from build123d import *

# Parameters (mm, degrees)
SKETCH1_R           = 2.0999999
BOSS_EXTRUDE1_DEPTH = 420


with BuildPart() as part:
    # Sketch1 → Boss-Extrude1 (new body)
    with BuildSketch(Plane.XY):
        with BuildLine():
            Line((-10, -13.3000005), (-10, -19))
            ThreePointArc((-10, -19), (-9.707106781, -19.707106781), (-9, -20))
            Line((-9, -20), (-3.3, -20))
            ThreePointArc((-3.3, -20), (-3.087867966, -19.912132034), (-3, -19.7))
            Line((-3, -19.7), (-3, -18))
            Line((-3, -18), (-6, -18))
            Line((-6, -18), (-6, -17.0606825))
            Line((-6, -17.0606825), (-2.939318, -14))
            Line((-2.939318, -14), (-0.519615242, -14))
            Line((-0.519615242, -14), (0, -13.7))
            Line((0, -13.7), (0.519615242, -14))
            Line((0.519615242, -14), (2.9393365, -14))
            Line((2.9393365, -14), (6, -17.0606628))
            Line((6, -17.0606628), (6, -18))
            Line((6, -18), (3, -18))
            Line((3, -18), (3, -19.7))
            ThreePointArc((3, -19.7), (3.087867966, -19.912132034), (3.3, -20))
            Line((3.3, -20), (9, -20))
            ThreePointArc((9, -20), (9.707106781, -19.707106781), (10, -19))
            Line((10, -19), (10, -13.3000005))
            ThreePointArc((10, -13.3000005), (9.912132034, -13.087868466), (9.7, -13.0000005))
            Line((9.7, -13.0000005), (8, -13.0000005))
            Line((8, -13.0000005), (8, -16.0000005))
            Line((8, -16.0000005), (7.06065685, -16.0000005))
            Line((7.06065685, -16.0000005), (4, -12.93934215))
            Line((4, -12.93934215), (4, -10.519615742))
            Line((4, -10.519615742), (3.7, -10.0000005))
            Line((3.7, -10.0000005), (4, -9.480385258))
            Line((4, -9.480385258), (4, -7.06068365))
            Line((4, -7.06068365), (7.06068236, -4.000000504))
            Line((7.06068236, -4.000000504), (8, -4.000000504))
            Line((8, -4.000000504), (8, -7.0000005))
            Line((8, -7.0000005), (9.7, -7.0000005))
            ThreePointArc((9.7, -7.0000005), (9.912132034, -6.912132534), (10, -6.7000005))
            Line((10, -6.7000005), (10, 6.7))
            ThreePointArc((10, 6.7), (9.912132034, 6.912132034), (9.7, 7))
            Line((9.7, 7), (8, 7))
            Line((8, 7), (8, 4))
            Line((8, 4), (7.060678, 4))
            Line((7.060678, 4), (4, 7.06068075))
            Line((4, 7.06068075), (4, 9.480384758))
            Line((4, 9.480384758), (3.7, 10))
            Line((3.7, 10), (4, 10.519615242))
            Line((4, 10.519615242), (4, 12.93933675))
            Line((4, 12.93933675), (7.060661, 16))
            Line((7.060661, 16), (8, 16))
            Line((8, 16), (8, 13))
            Line((8, 13), (9.7, 13))
            ThreePointArc((9.7, 13), (9.912132034, 13.087867966), (10, 13.3))
            Line((10, 13.3), (10, 19))
            ThreePointArc((10, 19), (9.707106781, 19.707106781), (9, 20))
            Line((9, 20), (3.3, 20))
            ThreePointArc((3.3, 20), (3.087867966, 19.912132034), (3, 19.7))
            Line((3, 19.7), (3, 18))
            Line((3, 18), (6, 18))
            Line((6, 18), (6, 17.06065975))
            Line((6, 17.06065975), (2.939354, 14))
            Line((2.939354, 14), (0.519638625, 14))
            Line((0.519638625, 14), (0, 13.6999865))
            Line((0, 13.6999865), (-0.519638625, 14))
            Line((-0.519638625, 14), (-2.939335, 14))
            Line((-2.939335, 14), (-6, 17.060678))
            Line((-6, 17.060678), (-6, 18))
            Line((-6, 18), (-3, 18))
            Line((-3, 18), (-3, 19.7))
            ThreePointArc((-3, 19.7), (-3.087867966, 19.912132034), (-3.3, 20))
            Line((-3.3, 20), (-9, 20))
            ThreePointArc((-9, 20), (-9.707106781, 19.707106781), (-10, 19))
            Line((-10, 19), (-10, 13.3))
            ThreePointArc((-10, 13.3), (-9.912132034, 13.087867966), (-9.7, 13))
            Line((-9.7, 13), (-8, 13))
            Line((-8, 13), (-8, 16))
            Line((-8, 16), (-7.060642, 16))
            Line((-7.060642, 16), (-4, 12.9393565))
            Line((-4, 12.9393565), (-4, 10.519615242))
            Line((-4, 10.519615242), (-3.7, 10))
            Line((-3.7, 10), (-4, 9.480384758))
            Line((-4, 9.480384758), (-4, 7.06066))
            Line((-4, 7.06066), (-7.060659, 4))
            Line((-7.060659, 4), (-8, 4))
            Line((-8, 4), (-8, 7))
            Line((-8, 7), (-9.7, 7))
            ThreePointArc((-9.7, 7), (-9.912132034, 6.912132034), (-10, 6.7))
            Line((-10, 6.7), (-10, -6.7000005))
            ThreePointArc((-10, -6.7000005), (-9.912132034, -6.912132534), (-9.7, -7.0000005))
            Line((-9.7, -7.0000005), (-8, -7.0000005))
            Line((-8, -7.0000005), (-8, -4.0000005))
            Line((-8, -4.0000005), (-7.06066257, -4.0000005))
            Line((-7.06066257, -4.0000005), (-4, -7.0606688))
            Line((-4, -7.0606688), (-4, -9.480385258))
            Line((-4, -9.480385258), (-3.7, -10.0000005))
            Line((-3.7, -10.0000005), (-4, -10.519615742))
            Line((-4, -10.519615742), (-4, -12.9393575))
            Line((-4, -12.9393575), (-7.0606365, -16.0000005))
            Line((-7.0606365, -16.0000005), (-8, -16.0000005))
            Line((-8, -16.0000005), (-8, -13.0000005))
            Line((-8, -13.0000005), (-9.7, -13.0000005))
            ThreePointArc((-9.7, -13.0000005), (-9.912132034, -13.087868466), (-10, -13.3000005))
        make_face()
        with Locations((0, 10)):
            Circle(SKETCH1_R, mode=Mode.SUBTRACT)
        with Locations((0, -10.0000005)):
            Circle(SKETCH1_R, mode=Mode.SUBTRACT)
        with BuildLine():
            Line((-8, 1.6999995), (-8, -1.70000025))
            ThreePointArc((-8, -1.70000025), (-7.912132034, -1.912132284), (-7.7, -2.00000025))
            Line((-7.7, -2.00000025), (-7.063604538, -2.00000025))
            ThreePointArc((-7.063604538, -2.00000025), (-6.948800316, -2.022823986), (-6.851481305, -2.087861995))
            Line((-6.851481305, -2.087861995), (-2.939335, -6))
            Line((-2.939335, -6), (2.93933195, -6))
            Line((2.93933195, -6), (6.851479294, -2.087861656))
            ThreePointArc((6.851479294, -2.087861656), (6.948799922, -2.022824212), (7.06360515, -2.00000025))
            Line((7.06360515, -2.00000025), (7.7, -2.00000025))
            ThreePointArc((7.7, -2.00000025), (7.912132034, -1.912132284), (8, -1.70000025))
            Line((8, -1.70000025), (8, 1.6999995))
            ThreePointArc((8, 1.6999995), (7.912132034, 1.912131534), (7.7, 1.9999995))
            Line((7.7, 1.9999995), (7.06359945, 1.9999995))
            ThreePointArc((7.06359945, 1.9999995), (6.9487942, 2.022823721), (6.851474147, 2.087862153))
            Line((6.851474147, 2.087862153), (2.9393355, 6))
            Line((2.9393355, 6), (-2.939339, 6))
            Line((-2.939339, 6), (-6.851476944, 2.087862556))
            ThreePointArc((-6.851476944, 2.087862556), (-6.948795311, 2.022823488), (-7.063599538, 1.9999995))
            Line((-7.063599538, 1.9999995), (-7.7, 1.9999995))
            ThreePointArc((-7.7, 1.9999995), (-7.912132034, 1.912131534), (-8, 1.6999995))
        make_face(mode=Mode.SUBTRACT)
    extrude(amount=-BOSS_EXTRUDE1_DEPTH)


solid = part.part
For this review, take the finished solid that the model builds, in its own axes (mm). Give positions to 0.01 mm unless a question says otherwise; leave off trailing zeros. Put each result on its own line as item: value. Start each with the question number.
(1) For pin 1 (1.9 mm diameter, centred on x = 1.5, z = -279.5, fed in from -Y); pin 2 (2.5 mm diameter, centred on y = 11.5, z = -257.5, fed in from -X); pin 3 (1.2 mm diameter, centred on y = 11.5, z = -193, fed in from +X), all flat-tipped, find the tip position at first contact; note any pin that passes through.
(2) Wall thickness on L1, parallel to Y at x = 0, z = -158; L2, parallel to Y at x = -8.5, z = -114; L3, parallel to X at y = 5, z = -275.5: over which ranges is each line inside the solid? List them lowest first.
(3) Add section A-A, the plane z = -290.5. Give the number of separate pieces and of enclosed holes in the cut face, then the cut area to 3 significant figures.
Result:
1. pin 1: stops at y = -14
1. pin 2: stops at x = -4
1. pin 3: stops at x = 4
2. L1: y = -13.7 to -12.1, -7.9 to -6, 6 to 7.9, 12.1 to 13.7
2. L2: y = -20 to -13, -7 to 7, 13 to 20
2. L3: x = -10 to -8, -6.06 to -3.94, 3.94 to 6.06, 8 to 10
3. separate pieces: 1
3. enclosed holes: 3
3. area: 324 mm^2
